```python
from build123d import *

# Parameters (mm, degrees)
SKETCH_1_R          = 6.5
SKETCH_1_R_2        = 3
EXTRUDE_1_DEPTH     = 2.5
SKETCH_2_R          = 5.716050362
SKETCH_2_R_2        = 4.24621305
CUT_EXTRUDE_1_DEPTH = 0.5


with BuildPart() as part:
    # 草图1 → 凸台-拉伸1 (new, symmetric)
    with BuildSketch(Plane.XY):
        Circle(SKETCH_1_R)
        Circle(SKETCH_1_R_2, mode=Mode.SUBTRACT)
    extrude(amount=EXTRUDE_1_DEPTH, both=True)

    # 草图2 → 切除-拉伸1 (cut)
    with BuildSketch(Plane(origin=(0, 0, -2.5), x_dir=(-1, 0, 0), z_dir=(0, 0, -1))):
        Circle(SKETCH_2_R)
        Circle(SKETCH_2_R_2, mode=Mode.SUBTRACT)
    cut_extrude_1 = extrude(amount=-CUT_EXTRUDE_1_DEPTH, mode=Mode.SUBTRACT)

    # 镜向1: 切除-拉伸1 across plane
    add(cut_extrude_1.mirror(Plane.XY), mode=Mode.SUBTRACT)


solid = part.part
```
For this review, take the finished solid that the model builds, in its own axes (mm). A direction names the side the tool comes from. Round coordinates to 2 decimals unless told otherwise and drop trailing zeros. Order: outer loops, then holes, each group sorted by start corner. A loop starts at its lowest first (then second) coordinate and runs counter-clockwise, first axis right, second up.
Q1. Wall thickness on line 1 (Y direction, x = 0, z = -2.05); line 2 (Y direction, x = 0, z = -0.55); line 3 (Y direction, x = 1.75, z = -2.2): over which ranges is each line inside the solid? List them lowest first.
Findings below:
line 1: y = -6.5 to -5.72, -4.25 to -3, 3 to 4.25, 5.72 to 6.5
line 2: y = -6.5 to -3, 3 to 6.5
line 3: y = -6.26 to -5.44, -3.87 to -2.44, 2.44 to 3.87, 5.44 to 6.26
Q2. Insertion check: P1, Ø3, axis at x = 4, z = -0.5, coming from the +Y side; P2, Ø3, axis at y = -3, z = -1, coming from the +X side. Each pin has a flat end and moves straight along its axis. Give the tip position at first contact, or say it passes through.
Findings below:
P1: stops at y = 6
P2: stops at x = 6.32
Q3. We need section A-A, the plane y = 0. Give the boundary of the cut face in (x, z).
Findings below:
outline: (-6.5, -2.5) - (-5.72, -2.5) - (-5.72, -2) - (-4.25, -2) - (-4.25, -2.5) - (-3, -2.5) - (-3, 2.5) - (-4.25, 2.5) - (-4.25, 2) - (-5.72, 2) - (-5.72, 2.5) - (-6.5, 2.5) - close; (3, -2.5) - (4.25, -2.5) - (4.25, -2) - (5.72, -2) - (5.72, -2.5) - (6.5, -2.5) - (6.5, 2.5) - (5.72, 2.5) - (5.72, 2) - (4.25, 2) - (4.25, 2.5) - (3, 2.5) - close
Q4. We need section D-D, the plane y = -4.5. Give the boundary of the cut face in (x, z).
Findings below:
outline: (-4.69, -2.5) - (-3.52, -2.5) - (-3.52, -2) - (3.52, -2) - (3.52, -2.5) - (4.69, -2.5) - (4.69, 2.5) - (3.52, 2.5) - (3.52, 2) - (-3.52, 2) - (-3.52, 2.5) - (-4.69, 2.5) - close
Q5. We need section C-C, the plane z = -0.35. Give the boundary of the cut face in (x, y), plus the area to 3 significant figures.
Findings below:
outline: circle Ø13 at (0, 0); hole circle Ø6 at (0, 0)
area: 104 mm2
Q6. Machinability: for faces 4 (the flat face through (0, -6, 2.5)), 5 (the flat face through (4, -2, -2)), 6 (the cylindrical face through (0.92, -4.145, 2.254)), which of the approach directions +Z, -Z, +X, -X, +Y, -Y give a long, thin tool a straight path to every point of the face, cutting with its end or side? Answer none if there is none.
Findings below:
face 4: +Z, +X, -X, +Y, -Y
face 5: -Z
face 6: +Z
Q7. Mouldability with a two-part tool opening along X and no side actions: class faces 1 (the cylindrical face through (-5.158, -3.955, 0.035)), 2 (the cylindrical face through (-5.45, 1.72, 2.25)), 3 (the flat face through (-3, -1, -2.5)) as pulls with the +X half, pulls with the -X half, needs draft (parallel to the pull), parting line crosses it, or undercut.
Findings below:
face 1: parting line crosses it
face 2: undercut
face 3: needs draft
